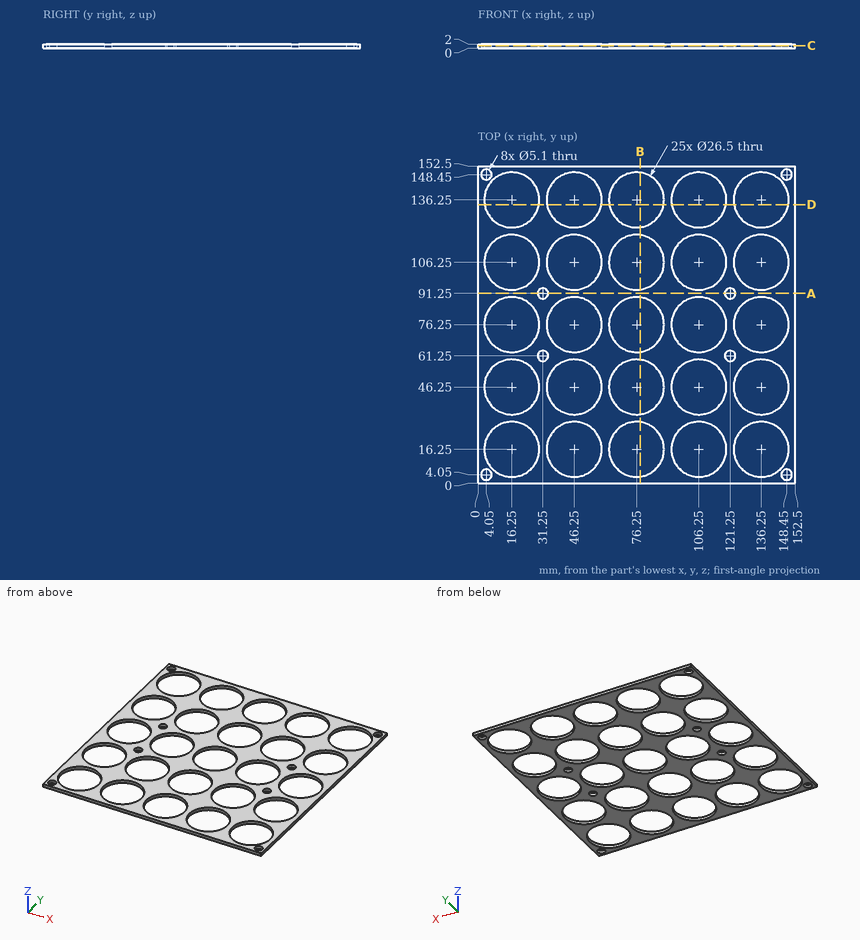
Geometry check sheet. Reference: drawing and pictorial views, mm from the part's lowest x, y, z. Round coordinates to 2 decimals unless told otherwise and drop trailing zeros. Order: outer loops, then holes, each group sorted by start corner. A loop starts at its lowest first (then second) coordinate and runs counter-clockwise, first axis right, second up. Notation, with made-up numbers: (-28, 73.25) -> (18, 73.25) arc R9 cw to (18, 79.25) -> close; hole circle Ø9 at (70.5, 83). An arc over 180 degrees is marked (long way). One line per item, written item: value. Start each with the question number.
Q1. Cross-section at D-D (y = 134). Record the boundary of the cut face in (x, z).
Q2. Thickness scan on line 1 (Y direction, x = 16.25, z = 0.95); line 2 (X direction, y = 49, z = 1.45); line 3 (Y direction, x = 28, z = 0.5). Record the ranges inside material, lowest first.
Q3. Cross-section at C-C (z = 1.2). Give the number of separate pieces and of enclosed holes in the cut face, and give its area (3 significant figures).
Q4. Cross-section at A-A (y = 91.25). Record the boundary of the cut face in (x, z).
Q5. Cross-section at B-B (x = 78). Record the boundary of the cut face in (y, z).
Completed:
1. outline: (0, 0) -> (3.19, 0) -> (3.19, 2) -> (0, 2) -> close; (29.31, 0) -> (33.19, 0) -> (33.19, 2) -> (29.31, 2) -> close; (59.31, 0) -> (63.19, 0) -> (63.19, 2) -> (59.31, 2) -> close; (89.31, 0) -> (93.19, 0) -> (93.19, 2) -> (89.31, 2) -> close; (119.31, 0) -> (123.19, 0) -> (123.19, 2) -> (119.31, 2) -> close; (149.31, 0) -> (152.5, 0) -> (152.5, 2) -> (149.31, 2) -> close
2. line 1: y = 0 to 3, 29.5 to 33, 59.5 to 63, 89.5 to 93, 119.5 to 123, 149.5 to 152.5
2. line 2: x = 0 to 3.29, 29.21 to 33.29, 59.21 to 63.29, 89.21 to 93.29, 119.21 to 123.29, 149.21 to 152.5
2. line 3: y = 0 to 10.13, 22.37 to 40.13, 52.37 to 70.13, 82.37 to 100.13, 112.37 to 130.13, 142.37 to 152.5
3. separate pieces: 1
3. enclosed holes: 33
3. area: 9,300 mm²
4. outline: (0, 0) -> (28.7, 0) -> (28.7, 2) -> (0, 2) -> close; (33.8, 0) -> (118.7, 0) -> (118.7, 2) -> (33.8, 2) -> close; (123.8, 0) -> (152.5, 0) -> (152.5, 2) -> (123.8, 2) -> close
5. outline: (0, 0) -> (3.12, 0) -> (3.12, 2) -> (0, 2) -> close; (29.38, 0) -> (33.12, 0) -> (33.12, 2) -> (29.38, 2) -> close; (59.38, 0) -> (63.12, 0) -> (63.12, 2) -> (59.38, 2) -> close; (89.38, 0) -> (93.12, 0) -> (93.12, 2) -> (89.38, 2) -> close; (119.38, 0) -> (123.12, 0) -> (123.12, 2) -> (119.38, 2) -> close; (149.38, 0) -> (152.5, 0) -> (152.5, 2) -> (149.38, 2) -> close
